Check sheet for the modelled part. Datum: model origin and axes. Units: mm. Give positions to 0.01 mm unless a question says otherwise; leave off trailing zeros. Order: outer loops, then holes, each group sorted by start corner. A loop starts at its lowest first (then second) coordinate and runs counter-clockwise, first axis right, second up. Notation, with made-up numbers: M 57,73.5 L 93,73.5 A16 ccw 93,79.5 Z; hole C 83.25,-39 d1. An arc over 180 degrees is marked long. Answer in a Markdown table with one row per item. Add a question column.
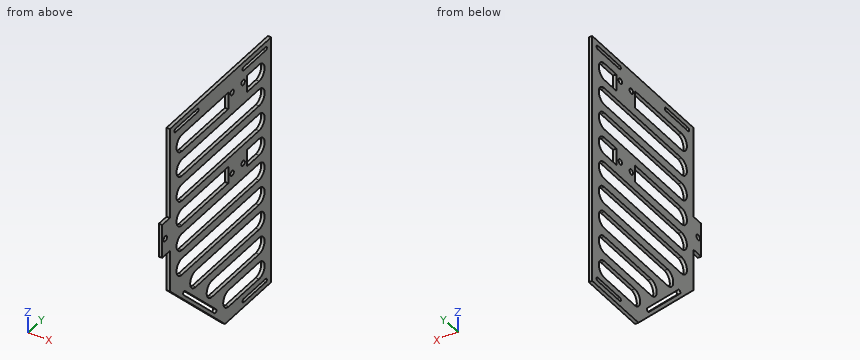
from build123d import *

# Parameters (mm, degrees)
SKETCH_2_W               = 148.55
SKETCH_2_H               = 92
EXTRUDE_1_DEPTH          = 2
CUT_EXTRUDE_1_DEPTH      = 88.388647003
CUT_EXTRUDE_1_DEPTH_BACK = 2
CUT_EXTRUDE_2_DEPTH      = 2
SKETCH_5_W               = 20
SKETCH_5_H               = 7
SKETCH_5_R               = 1.55
EXTRUDE_2_DEPTH          = 2
CUT_EXTRUDE_3_DEPTH      = 2
SKETCH_8_W               = 10
SKETCH_8_H               = 17
EXTRUDE_3_DEPTH          = 2
SKETCH_7_R               = 1.55
CUT_EXTRUDE_4_DEPTH      = 2
CUT_EXTRUDE_5_DEPTH      = 2


with BuildPart() as part:
    # 草图2 → 凸台-拉伸1 (new body)
    with BuildSketch(Plane(origin=(0, 0, 0), x_dir=(0, 0, -1), z_dir=(1, 0, 0))):
        Rectangle(SKETCH_2_W, SKETCH_2_H)
    extrude(amount=EXTRUDE_1_DEPTH)

    # 草图3 → 切除-拉伸1 (cut, two sides: drawn at the far end of the back side and taken through both)
    with BuildSketch(Plane(origin=(2, 0, 0), x_dir=(0, 0, -1), z_dir=(1, 0, 0)).offset(-CUT_EXTRUDE_1_DEPTH_BACK)):
        Polygon((-204.458434938, -274.733434938), (24.275, -46), (74.275, 4), (303.008434938, 232.733434938), (760.475304814, -224.733434938), (253.008434938, -732.200304814), align=None)
    extrude(amount=CUT_EXTRUDE_1_DEPTH + CUT_EXTRUDE_1_DEPTH_BACK, mode=Mode.SUBTRACT)

    # 草图4 → 切除-拉伸2 (cut)
    with BuildSketch(Plane(origin=(2, 0, 0), x_dir=(0, 0, -1), z_dir=(1, 0, 0))):
        with BuildLine():
            Line((-71.365, -41), (-71.365, -21))
            ThreePointArc((-71.365, -21), (-70.315, -19.95), (-69.265, -21))
            Line((-69.265, -21), (-69.265, -41))
            ThreePointArc((-69.265, -41), (-70.315, -42.05), (-71.365, -41))
        make_face()
        with BuildLine():
            Line((-71.365, 41), (-71.365, 21))
            ThreePointArc((-71.365, 21), (-70.315, 19.95), (-69.265, 21))
            Line((-69.265, 21), (-69.265, 41))
            ThreePointArc((-69.265, 41), (-70.315, 42.05), (-71.365, 41))
        make_face()
        with BuildLine():
            Line((71.365, 41), (71.365, 21))
            ThreePointArc((71.365, 21), (70.315, 19.95), (69.265, 21))
            Line((69.265, 21), (69.265, 41))
            ThreePointArc((69.265, 41), (70.315, 42.05), (71.365, 41))
        make_face()
    extrude(amount=-CUT_EXTRUDE_2_DEPTH, mode=Mode.SUBTRACT)

    # 草图5 → 凸台-拉伸2 (add)
    with BuildSketch(Plane(origin=(2, 0, 0), x_dir=(0, 0, -1), z_dir=(1, 0, 0))):
        with Locations((-10.315, -49.5)):
            Rectangle(SKETCH_5_W, SKETCH_5_H)
        with Locations((-10.315, -50.25)):
            Circle(SKETCH_5_R, mode=Mode.SUBTRACT)
    extrude(amount=-EXTRUDE_2_DEPTH)

    # 草图6 → 切除-拉伸3 (cut)
    with BuildSketch(Plane(origin=(2, 0, 0), x_dir=(0, 0, -1), z_dir=(1, 0, 0))):
        with BuildLine():
            Line((-64.275, -35), (-64.275, 35))
            ThreePointArc((-64.275, 35), (-59.275, 40), (-54.275, 35))
            Line((-54.275, 35), (-54.275, -35))
            ThreePointArc((-54.275, -35), (-59.275, -40), (-64.275, -35))
        make_face()
        with BuildLine():
            Line((-49.275, -35), (-49.275, 35))
            ThreePointArc((-49.275, 35), (-44.275, 40), (-39.275, 35))
            Line((-39.275, 35), (-39.275, -35))
            ThreePointArc((-39.275, -35), (-44.275, -40), (-49.275, -35))
        make_face()
        with BuildLine():
            Line((-34.275, -35), (-34.275, 35))
            ThreePointArc((-34.275, 35), (-29.275, 40), (-24.275, 35))
            Line((-24.275, 35), (-24.275, -35))
            ThreePointArc((-24.275, -35), (-29.275, -40), (-34.275, -35))
        make_face()
        with BuildLine():
            Line((-19.275, -35), (-19.275, 35))
            ThreePointArc((-19.275, 35), (-14.275, 40), (-9.275, 35))
            Line((-9.275, 35), (-9.275, -35))
            ThreePointArc((-9.275, -35), (-14.275, -40), (-19.275, -35))
        make_face()
        with BuildLine():
            Line((-4.275, -35), (-4.275, 35))
            ThreePointArc((-4.275, 35), (0.725, 40), (5.725, 35))
            Line((5.725, 35), (5.725, -35))
            ThreePointArc((5.725, -35), (0.725, -40), (-4.275, -35))
        make_face()
        with BuildLine():
            Line((10.725, -35), (10.725, 35))
            ThreePointArc((10.725, 35), (15.725, 40), (20.725, 35))
            Line((20.725, 35), (20.725, -35))
            ThreePointArc((20.725, -35), (15.725, -40), (10.725, -35))
        make_face()
        with BuildLine():
            Line((25.725, -22.579437252), (25.725, 35))
            ThreePointArc((25.725, 35), (30.725, 40), (35.725, 35))
            Line((35.725, 35), (35.725, -22.579437252))
            ThreePointArc((35.725, -22.579437252), (30.725, -27.579437252), (25.725, -22.579437252))
        make_face()
        with BuildLine():
            Line((40.725, -7.579437252), (40.725, 35))
            ThreePointArc((40.725, 35), (45.725, 40), (50.725, 35))
            Line((50.725, 35), (50.725, -7.579437252))
            ThreePointArc((50.725, -7.579437252), (45.725, -12.579437252), (40.725, -7.579437252))
        make_face()
        with BuildLine():
            Line((55.725, 7.420562748), (55.725, 35))
            ThreePointArc((55.725, 35), (60.725, 40), (65.725, 35))
            Line((65.725, 35), (65.725, 7.420562748))
            ThreePointArc((65.725, 7.420562748), (60.725, 2.420562748), (55.725, 7.420562748))
        make_face()
    extrude(amount=-CUT_EXTRUDE_3_DEPTH, mode=Mode.SUBTRACT)

    # 草图8 → 凸台-拉伸3 (add)
    with BuildSketch(Plane(origin=(2, 0, 0), x_dir=(0, 0, -1), z_dir=(1, 0, 0))):
        with Locations((-59.275, 15.5)):
            Rectangle(SKETCH_8_W, SKETCH_8_H)
        with Locations((-14.275, 15.5)):
            Rectangle(SKETCH_8_W, SKETCH_8_H)
    extrude(amount=-EXTRUDE_3_DEPTH)

    # 草图7 → 切除-拉伸4 (cut)
    with BuildSketch(Plane(origin=(2, 0, 0), x_dir=(0, 0, -1), z_dir=(1, 0, 0))):
        with Locations((-62.275, 10.5)):
            Circle(SKETCH_7_R)
        with Locations(Location((-13.275, 10.5, 0), (0, 0, 180))):
            Circle(SKETCH_7_R)
        with Locations((-13.275, 20.5)):
            Circle(SKETCH_7_R)
        with Locations(Location((-62.275, 20.5, 0), (0, 0, 180))):
            Circle(SKETCH_7_R)
    extrude(amount=-CUT_EXTRUDE_4_DEPTH, mode=Mode.SUBTRACT)

    # 草图9 → 切除-拉伸5 (cut)
    with BuildSketch(Plane(origin=(2, 0, 0), x_dir=(0, 0, -1), z_dir=(1, 0, 0))):
        with BuildLine():
            Line((32.269081912, -32.27835316), (60.55335316, -3.994081912))
            ThreePointArc((60.55335316, -3.994081912), (62.0382774, -3.994081912), (62.0382774, -5.479006153))
            Line((62.0382774, -5.479006153), (33.754006153, -33.7632774))
            ThreePointArc((33.754006153, -33.7632774), (32.269081912, -33.7632774), (32.269081912, -32.27835316))
        make_face()
    extrude(amount=-CUT_EXTRUDE_5_DEPTH, mode=Mode.SUBTRACT)


solid = part.part
Q1. Cross-section at A-A (y = -50.25). Record the boundary of the cut face in (x, z) (3 decimals).
Q2. Cross-section at B-B (z = 27.5). Record the boundary of the cut face in (x, y), and give its area (3 significant figures).
Q3. Go/stop test with flat-tipped pins: pin 1 (1 mm diameter, centred on x = 1, y = -21.5, fed in from -Z) (3 decimals); pin 2 (1 mm diameter, centred on x = 1, z = 45, fed in from -Y). Record where each tip stops, or that it passes through.
Q4. Cross-section at C-C (y = 30). State how many separate pieces and enclosed holes the cut face has, and give its area (3 significant figures).
Q5. Thickness scan on probe 1 along Y at (x, z) = (0.7, -1); probe 2 along Y at (x, z) = (0.8, -24); probe 3 along Y at (x, z) = (0.25, 13.5). Record the ranges inside material, lowest first.
Values follow:
| question | item | result |
|---|---|---|
| 1 | outline | M 0,0.315 L 2,0.315 L 2,8.765 L 0,8.765 Z; M 0,11.865 L 2,11.865 L 2,20.315 L 0,20.315 Z |
| 2 | outline | M 0,-46 L 2,-46 L 2,-39.67 L 0,-39.67 Z; M 0,39.67 L 2,39.67 L 2,46 L 0,46 Z |
| 2 | area | 25.3 mm² |
| 3 | pin 1 | z = -49.275 |
| 3 | pin 2 | y = -46 |
| 4 | separate pieces | 12 |
| 4 | enclosed holes | 0 |
| 4 | area | 109 mm² |
| 5 | probe 1 | -46 to -39.99, 39.99 to 46 |
| 5 | probe 2 | -46 to 46 |
| 5 | probe 3 | -53 to -39.94, 7 to 8.97, 12.03 to 18.97, 22.03 to 24, 39.94 to 46 |
